from build123d import *

# Parameters (mm, degrees)
SKETCH1_W           = 520
SKETCH1_H           = 350
BASE_FLANGE1_DEPTH  = 3.26
SKETCH6_R           = 3.25
CUT_EXTRUDE1_DEPTH  = 10
SKETCH7_R           = 3.25
CUT_EXTRUDE2_DEPTH  = 10
SKETCH9_W           = 140
SKETCH9_H           = 30
CUT_EXTRUDE3_DEPTH  = 6.35
CHAMFER1_SIZE       = 30
SKETCH10_R          = 2.5
CUT_EXTRUDE4_DEPTH  = 10
SKETCH11_R          = 2.25
SKETCH11_W          = 100
SKETCH11_H          = 200
CUT_EXTRUDE5_DEPTH  = 10
SKETCH12_W          = 100
SKETCH12_H          = 7.375
BOSS_EXTRUDE2_DEPTH = 3.26
FILLET1_R           = 10
SKETCH13_W          = 73.414309182
SKETCH13_H          = 40
CUT_EXTRUDE6_DEPTH  = 10
CHAMFER2_SIZE       = 10
SKETCH14_R          = 2.5
CUT_EXTRUDE7_DEPTH  = 10
CHAMFER3_SIZE       = 3


# Sheet-metal steps are written as plain solids
with BuildPart() as part:
    # Sketch1 → Base-Flange1 (new body)
    with BuildSketch(Plane(origin=(0, 0, 0), x_dir=(1, 0, 0), z_dir=(0, 1, 0))):
        with Locations((0, -175)):
            Rectangle(SKETCH1_W, SKETCH1_H)
    extrude(amount=-BASE_FLANGE1_DEPTH)

    # Sketch6 → Cut-Extrude1 (cut)
    with BuildSketch(Plane(origin=(0, 0, 0), x_dir=(1, 0, 0), z_dir=(0, 1, 0))):
        with Locations(Location((62.5, -14.9625, 0), (0, 0, 270))):
            Circle(SKETCH6_R)
        with Locations(Location((0, -14.9625, 0), (0, 0, 270))):
            Circle(SKETCH6_R)
        with Locations(Location((-62.5, -14.9625, 0), (0, 0, 270))):
            Circle(SKETCH6_R)
    extrude(amount=-CUT_EXTRUDE1_DEPTH, mode=Mode.SUBTRACT)

    # Sketch7 → Cut-Extrude2 (cut)
    with BuildSketch(Plane(origin=(0, 0, 0), x_dir=(1, 0, 0), z_dir=(0, 1, 0))):
        with Locations(Location((-223.749160028, -139.138800169, 0), (0, 0, 270))):
            Circle(SKETCH7_R)
        with Locations(Location((-223.749160028, -274.331266718, 0), (0, 0, 270))):
            Circle(SKETCH7_R)
        with Locations(Location((223.749160028, -274.331266718, 0), (0, 0, 90))):
            Circle(SKETCH7_R)
        with Locations(Location((223.749160028, -139.138800169, 0), (0, 0, 90))):
            Circle(SKETCH7_R)
    extrude(amount=-CUT_EXTRUDE2_DEPTH, mode=Mode.SUBTRACT)

    # Sketch9 → Cut-Extrude3 (cut)
    with BuildSketch(Plane(origin=(0, 0, 0), x_dir=(1, 0, 0), z_dir=(0, 1, 0))):
        with Locations((0, -335)):
            Rectangle(SKETCH9_W, SKETCH9_H)
    extrude(amount=-CUT_EXTRUDE3_DEPTH, mode=Mode.SUBTRACT)

    # Chamfer1
    chamfer1_edges = [part.edges().sort_by_distance(p)[0] for p in [
        (260, -1.63, 350),
        (-260, -1.63, 350),
        (70, -1.63, 350),
        (-70, -1.63, 350),
    ]]
    chamfer(chamfer1_edges, length=CHAMFER1_SIZE - 0.0001)  # a hair under: the kernel refuses the full size

    # Sketch10 → Cut-Extrude4 (cut)
    with BuildSketch(Plane(origin=(0, 0, 0), x_dir=(1, 0, 0), z_dir=(0, 1, 0))):
        with Locations(Location((-52.5, -97.5, 0), (0, 0, 270))):
            Circle(SKETCH10_R)
        with Locations(Location((52.5, -97.5, 0), (0, 0, 270))):
            Circle(SKETCH10_R)
        with Locations(Location((52.5, -202.5, 0), (0, 0, 270))):
            Circle(SKETCH10_R)
        with Locations(Location((-52.5, -202.5, 0), (0, 0, 270))):
            Circle(SKETCH10_R)
        with BuildLine():
            Line((-3, -209.924953066), (-3, -169.773719933))
            ThreePointArc((-3, -169.773719933), (-7.653668647, -168.47759065), (-11.860811111, -166.103451798))
            Line((-11.860811111, -166.103451798), (-40.252020332, -194.494661019))
            ThreePointArc((-40.252020332, -194.494661019), (-22.961005942, -205.432771951), (-3, -209.924953066))
        make_face()
        with BuildLine():
            Line((-3, -90.075046934), (-3, -130.226280067))
            ThreePointArc((-3, -130.226280067), (-7.653668647, -131.52240935), (-11.860811111, -133.896548202))
            Line((-11.860811111, -133.896548202), (-40.252020332, -105.505338981))
            ThreePointArc((-40.252020332, -105.505338981), (-22.961005942, -94.567228049), (-3, -90.075046934))
        make_face()
        with BuildLine():
            Line((-19.773719933, -147), (-59.924953066, -147))
            ThreePointArc((-59.924953066, -147), (-55.432771951, -127.038994058), (-44.494661019, -109.747979668))
            Line((-44.494661019, -109.747979668), (-16.103451798, -138.139188889))
            ThreePointArc((-16.103451798, -138.139188889), (-18.47759065, -142.346331353), (-19.773719933, -147))
        make_face()
        with BuildLine():
            Line((-19.773719933, -153), (-59.924953066, -153))
            ThreePointArc((-59.924953066, -153), (-55.432771951, -172.961005942), (-44.494661019, -190.252020332))
            Line((-44.494661019, -190.252020332), (-16.103451798, -161.860811111))
            ThreePointArc((-16.103451798, -161.860811111), (-18.47759065, -157.653668647), (-19.773719933, -153))
        make_face()
        with BuildLine():
            Line((3, -209.924953066), (3, -169.773719933))
            ThreePointArc((3, -169.773719933), (7.653668647, -168.47759065), (11.860811111, -166.103451798))
            Line((11.860811111, -166.103451798), (40.252020332, -194.494661019))
            ThreePointArc((40.252020332, -194.494661019), (22.961005942, -205.432771951), (3, -209.924953066))
        make_face()
        with BuildLine():
            Line((44.494661019, -190.252020332), (16.103451798, -161.860811111))
            ThreePointArc((16.103451798, -161.860811111), (18.47759065, -157.653668647), (19.773719933, -153))
            Line((19.773719933, -153), (59.924953066, -153))
            ThreePointArc((59.924953066, -153), (55.432771951, -172.961005942), (44.494661019, -190.252020332))
        make_face()
        with BuildLine():
            Line((19.773719933, -147), (59.924953066, -147))
            ThreePointArc((59.924953066, -147), (55.432771951, -127.038994058), (44.494661019, -109.747979668))
            Line((44.494661019, -109.747979668), (16.103451798, -138.139188889))
            ThreePointArc((16.103451798, -138.139188889), (18.47759065, -142.346331353), (19.773719933, -147))
        make_face()
        with BuildLine():
            Line((40.252020332, -105.505338981), (11.860811111, -133.896548202))
            ThreePointArc((11.860811111, -133.896548202), (7.653668647, -131.52240935), (3, -130.226280067))
            Line((3, -130.226280067), (3, -90.075046934))
            ThreePointArc((3, -90.075046934), (22.961005942, -94.567228049), (40.252020332, -105.505338981))
        make_face()
    extrude(amount=-CUT_EXTRUDE4_DEPTH, mode=Mode.SUBTRACT)

    # Sketch11 → Cut-Extrude5 (cut)
    with BuildSketch(Plane(origin=(0, 0, 0), x_dir=(1, 0, 0), z_dir=(0, 1, 0))):
        with Locations(Location((-195, -265, 0), (0, 0, 270))):
            Circle(SKETCH11_R)
        with Locations(Location((-195, -55, 0), (0, 0, 270))):
            Circle(SKETCH11_R)
        with Locations(Location((-85, -55, 0), (0, 0, 270))):
            Circle(SKETCH11_R)
        with Locations(Location((-85, -265, 0), (0, 0, 270))):
            Circle(SKETCH11_R)
        with Locations(Location((-85, -160, 0), (0, 0, 270))):
            Circle(SKETCH11_R)
        with Locations(Location((-195, -160, 0), (0, 0, 270))):
            Circle(SKETCH11_R)
        with Locations(Location((195, -160, 0), (0, 0, 270))):
            Circle(SKETCH11_R)
        with Locations(Location((85, -160, 0), (0, 0, 270))):
            Circle(SKETCH11_R)
        with Locations(Location((85, -265, 0), (0, 0, 270))):
            Circle(SKETCH11_R)
        with Locations(Location((85, -55, 0), (0, 0, 270))):
            Circle(SKETCH11_R)
        with Locations(Location((195, -55, 0), (0, 0, 270))):
            Circle(SKETCH11_R)
        with Locations(Location((195, -265, 0), (0, 0, 270))):
            Circle(SKETCH11_R)
        with Locations((-140, -160)):
            Rectangle(SKETCH11_W, SKETCH11_H)
        with Locations((140, -160)):
            Rectangle(SKETCH11_W, SKETCH11_H)
    extrude(amount=-CUT_EXTRUDE5_DEPTH, mode=Mode.SUBTRACT)

    # Sketch12 → Boss-Extrude2 (add)
    with BuildSketch(Plane(origin=(0, 0, 0), x_dir=(1, 0, 0), z_dir=(0, 1, 0))):
        with Locations((-140, -133.068919425)):
            Rectangle(SKETCH12_W, SKETCH12_H)
    extrude(amount=-BOSS_EXTRUDE2_DEPTH)

    # Fillet1
    fillet1_edges = [part.edges().sort_by_distance(p)[0] for p in [
        (-90, -1.63, 60),
        (-90, -1.63, 260),
        (-190, -1.63, 260),
        (-190, -1.63, 60),
        (190, -1.63, 60),
        (190, -1.63, 260),
        (90, -1.63, 260),
        (90, -1.63, 60),
        (-190, -1.63, 136.756419425),
        (-190, -1.63, 129.381419425),
        (-90, -1.63, 129.381419425),
        (-90, -1.63, 136.756419425),
    ]]
    fillet(fillet1_edges, radius=FILLET1_R)

    # Sketch13 → Cut-Extrude6 (cut)
    with BuildSketch(Plane(origin=(0, 0, 0), x_dir=(1, 0, 0), z_dir=(0, 1, 0))):
        with Locations((0, -255)):
            Rectangle(SKETCH13_W, SKETCH13_H)
    extrude(amount=-CUT_EXTRUDE6_DEPTH, mode=Mode.SUBTRACT)

    # Chamfer2
    chamfer2_edges = [part.edges().sort_by_distance(p)[0] for p in [
        (36.707154591, -1.63, 235),
        (36.707154591, -1.63, 275),
        (-36.707154591, -1.63, 275),
        (-36.707154591, -1.63, 235),
    ]]
    chamfer(chamfer2_edges, length=CHAMFER2_SIZE)

    # Sketch14 → Cut-Extrude7 (cut)
    with BuildSketch(Plane(origin=(0, 0, 0), x_dir=(1, 0, 0), z_dir=(0, 1, 0))):
        with Locations(Location((-36.707154591, -275, 0), (0, 0, 270))):
            Circle(SKETCH14_R)
        with Locations(Location((-36.707154591, -235, 0), (0, 0, 270))):
            Circle(SKETCH14_R)
        with Locations(Location((36.707154591, -235, 0), (0, 0, 270))):
            Circle(SKETCH14_R)
        with Locations(Location((36.707154591, -275, 0), (0, 0, 270))):
            Circle(SKETCH14_R)
    extrude(amount=-CUT_EXTRUDE7_DEPTH, mode=Mode.SUBTRACT)

    # Chamfer3
    chamfer3_edges = [part.edges().sort_by_distance(p)[0] for p in [
        (62.5, 0, 11.7125),
        (0, 0, 11.7125),
        (-62.5, 0, 11.7125),
        (-223.749160028, 0, 135.888800169),
        (-223.749160028, 0, 271.081266718),
        (223.749160028, 0, 277.581266718),
        (223.749160028, 0, 142.388800169),
    ]]
    chamfer(chamfer3_edges, length=CHAMFER3_SIZE)


solid = part.part
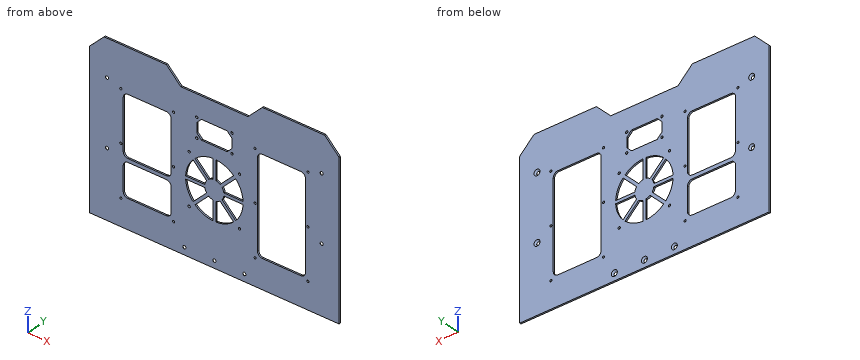
Geometry: final body of the model. Coordinates: model frame, mm. Give positions to 0.01 mm unless a question says otherwise; leave off trailing zeros. Write each loop counter-clockwise with the first axis right and the second up, starting at its lowest first coordinate (ties: lowest second). Pieces come first, ordered by that corner, then holes. Notation, with made-up numbers: M -34.75,80 L -30.75,80 A18 ccw -30.75,89 Z; hole C 72.25,46.25 d6. An arc over 180 degrees is marked long. Answer in a Markdown table with one row per item. Add a question column.
(1) Section D-D on z = 176.5. Return loops of the section in (x, y), and give its area (3 significant figures).
(2) Section B-B on x = 168. Return loops of the section in (y, z).
(3) Section C-C on x = -113. Return loops of the section in (y, z).
(4) Section A-A on z = 216. Return loops of the section in (x, y), and give its area (3 significant figures).
(5) Ray query, line 1 (Z direction, x = -105, y = -0.4); line 2 (X direction, y = -2.45, z = 55); line 3 (Z direction, x = 195, y = -0.85). Return the intervals inside material, ascending.
(6) First-contact query: pin 1 (8.5 mm diameter, centred on x = 0, z = 14.96, fed in from +Y); pin 2 (5 mm diameter, centred on x = -223.75, z = 139.14, fed in from +Y); pin 3 (1.6 mm diameter, centred on x = -30.5, y = -1, fed in from +Z). Flat tips, straight axial feed; report the tip coordinate or a pass-through.
Result set:
| question | item | result |
|---|---|---|
| 1 | outline | M -260,-3.26 L -190,-3.26 L -190,0 L -260,0 Z; M -90,-3.26 L -53.83,-3.26 L -53.83,0 L -90,0 Z; M -30.74,-3.26 L -22.26,-3.26 L -22.26,0 L -30.74,0 Z; M -3,-3.26 L 3,-3.26 L 3,0 L -3,0 Z; M 22.26,-3.26 L 30.74,-3.26 L 30.74,0 L 22.26,0 Z; M 53.83,-3.26 L 90,-3.26 L 90,0 L 53.83,0 Z; M 190,-3.26 L 260,-3.26 L 260,0 L 190,0 Z |
| 1 | area | 767 mm^2 |
| 2 | outline | M -3.26,0 L 0,0 L 0,60 L -3.26,60 Z; M -3.26,260 L 0,260 L 0,350 L -3.26,350 Z |
| 3 | outline | M -3.26,0 L 0,0 L 0,60 L -3.26,60 Z; M -3.26,129.38 L 0,129.38 L 0,136.76 L -3.26,136.76 Z; M -3.26,260 L 0,260 L 0,350 L -3.26,350 Z |
| 4 | outline | M -260,-3.26 L -190,-3.26 L -190,0 L -260,0 Z; M -90,-3.26 L 90,-3.26 L 90,0 L -90,0 Z; M 190,-3.26 L 260,-3.26 L 260,0 L 190,0 Z |
| 4 | area | 1,040 mm^2 |
| 5 | line 1 | z = 0 to 60, 129.38 to 136.76, 260 to 350 |
| 5 | line 2 | x = -260 to -197.25, -192.75 to -87.25, -82.75 to 82.75, 87.25 to 192.75, 197.25 to 260 |
| 5 | line 3 | z = 0 to 52.75, 57.25 to 157.75, 162.25 to 262.75, 267.25 to 350 |
| 6 | pin 1 | stops at y = -2 |
| 6 | pin 2 | passes through |
| 6 | pin 3 | stops at z = 320 |
